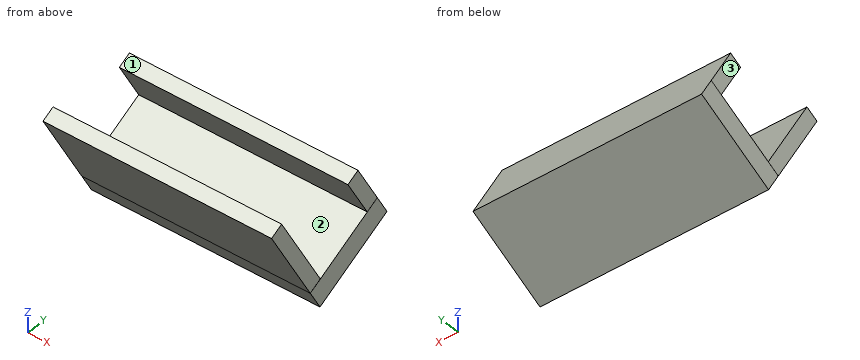
from build123d import *

# Parameters (mm, degrees)
SKETCH051_W             = 50
SKETCH051_H             = 20
PAD050_DEPTH            = 5
SKETCH052_W             = 50
SKETCH052_H             = 3
PAD051_DEPTH            = 20
SKETCH053_W             = 50
SKETCH053_H             = 10
PAD052_DEPTH            = 3
BODY041_PLACEMENT_ANGLE = 30


with BuildPart() as part:
    # Sketch051 → Pad050 (new body)
    with BuildSketch(Plane.XY):
        with Locations((184.845276, -123.914059)):
            Rectangle(SKETCH051_W, SKETCH051_H)
    extrude(amount=PAD050_DEPTH)

    # Sketch052 (on Face6 of Pad050) → Pad051 (join)
    with BuildSketch(Plane.XY.offset(5)):
        with Locations((184.83606, -132.417099)):
            Rectangle(SKETCH052_W, SKETCH052_H)
    extrude(amount=PAD051_DEPTH)

    # Sketch053 (on Face7 of Pad051) → Pad052 (join)
    with BuildSketch(Plane(origin=(0, -113.914059, 0), x_dir=(-1, 0, 0), z_dir=(0, 1, 0))):
        with Locations((-184.841869, 9.989668)):
            Rectangle(SKETCH053_W, SKETCH053_H)
    extrude(amount=-PAD052_DEPTH)


with BuildPart() as part_1:
    # Body041 placement: moved
    add(part.part.moved(Location((-180.1, 172.766257, 123.466258))).rotate(Axis((-180.1, 172.766257, 123.466258), (1, 0, 0)), BODY041_PLACEMENT_ANGLE))


solid = part_1.part
The listing builds one solid part. Answer for the finished solid, in the listing's coordinates (mm). Face numbers are marked on the shaded views. A direction names the side the tool comes from. Coordinates: 2 decimals unless noted, no trailing zeros. Order: outer loops, then holes, each group sorted by start corner. A loop starts at its lowest first (then second) coordinate and runs counter-clockwise, first axis right, second up.
Q1. Which of the six approach directions +Z, -Z, +X, -X, +Y, -Y give full straight-line access (tool end or side, diameter ignored) to the marked faces 1, 2 and 3?
Q2. A cutting plane is placed at A-A, the plane y = 67.75. Write down the section's boundary in (x, z).
Q3. A cutting plane is placed at B-B, the plane z = 77. Write down the section's boundary in (x, y), and give its area (3 significant figures).
Q4. Given P1, Ø1.5, axis at y = 68, z = 71, coming from the -X side; P2, Ø12, axis at x = 14, z = 63.5, coming from the -Y side; P3, Ø1, axis at x = -3.5, z = 68, coming from the +Y side, each flat-ended and moving along its own axis, determine where each tip first touches the part or whether it passes through.
Q5. A cutting plane is placed at D-D, the plane z = 58.75. Write down the section's boundary in (x, y).
Q6. Consider line 1 (X direction, y = 72.75, z = 67); line 2 (Y direction, x = -6, z = 69.75); line 3 (Y direction, x = -1.5, z = 66). Determine where each line is inside the solid, lowest interval first.
Answers follow:
1. face 1: +Z, +X, -X
1. face 2: +X, -X
1. face 3: +Z, -Z, -X, +Y, -Y
2. outline: (-20.26, 71.53) - (29.74, 71.53) - (29.74, 77.53) - (-20.26, 77.53) - close; (-20.25, 62.84) - (29.75, 62.84) - (29.75, 68.61) - (-20.25, 68.61) - close
3. outline: (-20.26, 44.96) - (29.74, 44.96) - (29.74, 48.42) - (-20.26, 48.42) - close; (-20.26, 64.59) - (29.74, 64.59) - (29.74, 68.06) - (-20.26, 68.06) - close
3. area: 346 mm2
4. P1: stops at x = -20.26
4. P2: stops at y = 49.29
4. P3: stops at y = 73.54
5. outline: (-20.25, 55.5) - (29.75, 55.5) - (29.75, 60.67) - (-20.25, 60.67) - close
6. line 1: x = -20.25 to 29.75
6. line 2: y = 49.15 to 52.61, 68.78 to 72.24
6. line 3: y = 51.31 to 54.77, 63.23 to 73.23
